CAD build for the part. Positions are in the model's coordinates, mm. A direction names the side the tool comes from. Coordinates: 2 decimals unless noted, no trailing zeros. Order: outer loops, then holes, each group sorted by start corner. A loop starts at its lowest first (then second) coordinate and runs counter-clockwise, first axis right, second up. Notation, with made-up numbers: M -24,73.25 L -19,73.25 A15 cw -19,99.25 Z; hole C 29.25,44.5 d1. An arc over 180 degrees is marked long. Write item = value, one per line.
Autodesk Inventor part; units mm, degrees
ref_plane "YZ Plane" through (0, 0, 0) normal (1, 0, 0) x (0, 1, 0)
ref_plane "XZ Plane" through (0, 0, 0) normal (0, 1, 0) x (-1, 0, 0)
ref_plane "XY Plane" through (0, 0, 0) normal (0, 0, 1) x (1, 0, 0)
sketch "Sketch1" plane through (0, 0, 0) normal (0, 1, 0) x (-1, 0, 0)
  line L0 (18, 20) -> (-18, 20)
  line L1 (-20, 18) -> (-20, -18)
  line L2 (-18, -20) -> (18, -20)
  line L3 (20, -18) -> (20, 18)
  line L4 (20, 20) -> (-20, -20) construction
  line L5 (-20, 20) -> (20, -20) construction
  circle A0 centre (0, 0) radius 11.5
  circle A1 centre (0, 0) radius 18.945
  arc A2 (20, 18) -> (18, 20) centre (18, 18) ccw
  arc A3 (18, -20) -> (20, -18) centre (18, -18) ccw
  arc A4 (-20, -18) -> (-18, -20) centre (-18, -18) ccw
  arc A5 (-18, 20) -> (-20, 18) centre (-18, 18) ccw
  dimension "d0" = 40
  dimension "d1" = 40
  dimension "d2" = 23
  dimension "d3" = 37.89
  dimension "d4" = 2
extrude "Extrusion1" add sketch "Sketch1" along normal blind 11
sketch "Sketch2" plane through (0, 0, 0) normal (0, -1, 0) x (1, 0, 0)
  line L0 (-20, -18) -> (-20, 18)
  arc A0 (-18, 20) -> (-20, 18) centre (-18, 18) ccw
  line L1 (-18, 20) -> (18, 20)
  arc A1 (20, 18) -> (18, 20) centre (18, 18) ccw
  line L2 (20, 18) -> (20, -18)
  arc A2 (18, -20) -> (20, -18) centre (18, -18) ccw
  line L3 (18, -20) -> (-18, -20)
  arc A3 (-20, -18) -> (-18, -20) centre (-18, -18) ccw
  point P0 (0, 0)
extrude "Extrusion2" add sketch "Sketch2" against normal blind 1
sketch "Sketch3" plane through (0, 11, 0) normal (0, 1, 0) x (1, 0, 0)
  circle A0 centre (0, 0) radius 11.5
  circle A1 centre (0, 0) radius 10.9
  dimension "d9" = 0.6
extrude "Extrusion3" cut sketch "Sketch3" against normal through all contours A1
sketch "Sketch4" plane through (0, 11, 0) normal (0, 1, 0) x (1, 0, 0)
  circle A0 centre (0, 0) radius 18.945 construction
  line L0 (-18, -20) -> (18, -20) construction
  arc A1 (18, -20) -> (20, -18) centre (18, -18) ccw construction
  line L1 (20, -18) -> (20, 18) construction
  arc A2 (20, 18) -> (18, 20) centre (18, 18) ccw construction
  line L2 (18, 20) -> (-18, 20) construction
  arc A3 (-18, 20) -> (-20, 18) centre (-18, 18) ccw construction
  line L3 (-20, 18) -> (-20, -18) construction
  arc A4 (-20, -18) -> (-18, -20) centre (-18, -18) ccw construction
  line L4 (-16.1, -16.1) -> (16.1, -16.1) construction
  line L5 (16.1, -16.1) -> (16.1, 16.1) construction
  line L6 (16.1, 16.1) -> (-16.1, 16.1) construction
  line L7 (-16.1, 16.1) -> (-16.1, -16.1) construction
  line L8 (-16.1, -16.1) -> (16.1, 16.1) construction
  line L9 (16.1, -16.1) -> (-16.1, 16.1) construction
  point P0 (0, 0)
  dimension "d12" = 32.2
  dimension "d13" = 32.2
hole "Hole1" at (-16.1, 11, 16.1) at (-16.1, 11, -16.1) at (16.1, 11, -16.1) at (16.1, 11, 16.1) direction (0, -1, 0) diameter 3.85 depth 10
sketch "Sketch14" plane through (20, 0, -18) normal (1, 0, 0) x (0, 0, -1)
  line L0 (0, 0) -> (0, 11) construction
  line L1 (-36, 11) -> (0, 11) construction
  line L2 (-36, 0) -> (-36, 11) construction
  line L3 (-36, 0) -> (0, 0) construction
  line L4 (-25.5, 10) -> (-10.5, 10)
  line L5 (-10.5, 10) -> (-10.5, 1)
  line L6 (-10.5, 1) -> (-25.5, 1)
  line L7 (-25.5, 1) -> (-25.5, 10)
  line L8 (-25.5, 10) -> (-10.5, 1) construction
  line L9 (-10.5, 10) -> (-25.5, 1) construction
  point P0 (-18, 0)
  point P1 (-18, 5.5)
  dimension "d47" = 15
  dimension "d48" = 9
extrude "Extrusion12" cut sketch "Sketch14" against normal blind 3
fillet "Fillet2" radius 2 2 edges at (17.3972, 5.5, 7.5) (17.3972, 5.5, -7.5)
sketch "Sketch15" plane through (0, 1, 0) normal (0, 1, 0) x (1, 0, 0)
  arc A0 (18.6666, -7.5) -> (16.8842, -8.5929) centre (18.6666, -9.5) ccw construction
  line L0 (20, -7.5) -> (18.6666, -7.5) construction
  line L1 (20, 7.5) -> (20, -7.5) construction
  line L2 (20, 7.5) -> (18.6666, 7.5) construction
  arc A1 (16.8842, 8.5929) -> (18.6666, 7.5) centre (18.6666, 9.5) ccw construction
  arc A2 (16.6035, -9.1235) -> (16.8842, -8.5929) centre (0, 0) ccw
  arc A3 (11.2223, -2.5118) -> (11.5, 0.0176) centre (0, 0) ccw
  arc A4 (11.5, 0.0176) -> (16.8842, -8.5929) centre (21.1006, 0.0323) ccw
  arc A5 (10.9, 0.0167) -> (16.6207, -9.1319) centre (21.1006, 0.0323) ccw
  dimension "d52" = 0.6
extrude "Extrusion13" add sketch "Sketch15" along normal up to surface (10 mm away)
sketch "Sketch16" plane through (20, 10, -7.5) normal (0, -1, 0) x (1, 0, 0)
  arc A0 (-3.1158, -1.0929) -> (-3.1158, 16.0929) centre (-20, 7.5) ccw
  arc A1 (-1.3334, 0) -> (-3.1158, -1.0929) centre (-1.3334, -2) ccw
  line L0 (0, 0) -> (-1.3334, 0)
  line L1 (0, 15) -> (0, 0)
  line L2 (0, 15) -> (-1.3334, 15)
  arc A2 (-3.1158, 16.0929) -> (-1.3334, 15) centre (-1.3334, 17) ccw
extrude "Extrusion14" add sketch "Sketch16" along normal up to surface (9 mm away)
sketch "Sketch17" plane through (20, 0, -18) normal (1, 0, 0) x (0, 0, -1)
  line L0 (0, 0) -> (0, 11) construction
  line L1 (-36, 11) -> (0, 11) construction
  line L2 (-36, 0) -> (-36, 11) construction
  line L3 (-36, 0) -> (0, 0) construction
  circle A0 centre (-17.9824, 5.5) radius 5.1
  point P0 (-18, 0)
  dimension "d57" = 10.2
extrude "Extrusion15" cut sketch "Sketch17" against normal blind 3
sketch "Sketch18" plane through (0, 11, 0) normal (0, 1, 0) x (1, 0, 0)
  line L0 (-18, -20) -> (18, -20)
  arc A0 (18, -20) -> (20, -18) centre (18, -18) ccw
  line L1 (20, -18) -> (20, 18)
  arc A1 (20, 18) -> (18, 20) centre (18, 18) ccw
  line L2 (18, 20) -> (-18, 20)
  arc A2 (-18, 20) -> (-20, 18) centre (-18, 18) ccw
  line L3 (-20, 18) -> (-20, -18)
  arc A3 (-20, -18) -> (-18, -20) centre (-18, -18) ccw
  circle A4 centre (16.1, -16.1) radius 1.925
  circle A5 centre (-16.1, 16.1) radius 1.925
  circle A6 centre (-16.1, -16.1) radius 1.925
  circle A7 centre (16.1, 16.1) radius 1.925
  circle A8 centre (0, 0) radius 10.9
  arc A9 (11.5, 0.0176) -> (11.2223, -2.5118) centre (0, 0) ccw
  arc A10 (11.2223, -2.5118) -> (16.6035, -9.1235) centre (21.1006, 0.0323) ccw
  arc A11 (16.8842, -8.5929) -> (16.6035, -9.1235) centre (0, 0) ccw
  arc A12 (11.5, 0.0176) -> (16.8842, -8.5929) centre (21.1006, 0.0323) ccw
extrude "Extrusion16" add sketch "Sketch18" along normal blind 1
sketch "Sketch19" plane through (0, 0, 0) normal (0, 1, 0) x (-1, 0, 0)
  arc A0 (-11.2223, 2.5118) -> (-16.6035, 9.1235) centre (-21.1006, -0.0323) ccw construction
  arc A1 (-16.8842, 8.5929) -> (-16.6035, 9.1235) centre (0, 0) ccw construction
  arc A2 (-11.5, -0.0176) -> (-16.8842, 8.5929) centre (-21.1006, -0.0323) ccw construction
  arc A3 (-11.5, -0.0176) -> (-11.2223, 2.5118) centre (0, 0) ccw construction
  circle A4 centre (0, 0) radius 10.9 construction
  circle A5 centre (-16.1, -16.1) radius 1.925 construction
  circle A6 centre (16.1, 16.1) radius 1.925 construction
  circle A7 centre (16.1, -16.1) radius 1.925 construction
  circle A8 centre (-16.1, 16.1) radius 1.925 construction
  line L0 (18, 20) -> (-18, 20) construction
  arc A9 (-18, 20) -> (-20, 18) centre (-18, 18) ccw construction
  line L1 (-20, 18) -> (-20, -18) construction
  arc A10 (-20, -18) -> (-18, -20) centre (-18, -18) ccw construction
  line L2 (-18, -20) -> (18, -20) construction
  arc A11 (18, -20) -> (20, -18) centre (18, -18) ccw construction
  line L3 (20, -18) -> (20, 18) construction
  arc A12 (20, 18) -> (18, 20) centre (18, 18) ccw construction
sketch "Sketch5" plane through (20, 0, -18) normal (1, 0, 0) x (0, 0, -1)
  line L0 (0, 0) -> (0, 11) construction
  line L1 (-36, 11) -> (0, 11) construction
  line L2 (-36, 0) -> (-36, 11) construction
  line L3 (-36, 0) -> (0, 0) construction
  line L4 (-20.5, 10) -> (-5.5, 10)
  line L5 (-5.5, 10) -> (-5.5, 1)
  line L6 (-5.5, 1) -> (-20.5, 1)
  line L7 (-20.5, 1) -> (-20.5, 10)
  line L8 (-20.5, 10) -> (-5.5, 1) construction
  line L9 (-5.5, 10) -> (-20.5, 1) construction
  point P0 (-18, 0)
  point P1 (-13, 5.5)
  dimension "d21" = 15
  dimension "d22" = 9
sketch "Sketch6" plane through (0, 1, 0) normal (0, 1, 0) x (1, 0, 0)
  line L0 (20, -2.5) -> (18.7339, -2.5) construction
  arc A0 (15.4996, 2.2947) -> (15.8884, 4.3911) centre (6.7587, 5) ccw
  arc A1 (15.8884, 4.3911) -> (18.7339, -2.5) centre (25.6093, 4.3721) ccw
  arc A2 (15.4996, 2.2947) -> (18.3979, -3.0115) centre (25.6093, 4.3721) ccw
  arc A3 (18.3979, -3.0115) -> (18.7339, -2.5) centre (6.7587, 5) ccw
  arc A4 (18.3979, -3.0115) -> (18.7339, -2.5) centre (6.7587, 5) ccw
  point P0 (0, 0)
  dimension "d25" = 0.6
sketch "Sketch12" plane through (20, 10, -12.5) normal (0, -1, 0) x (1, 0, 0)
  arc A0 (-4, 2.4397) -> (-1.2661, 15) centre (-20, 12.5) ccw
  line L0 (0, 0) -> (-4, 0)
  line L1 (0, 15) -> (0, 0)
  line L2 (0, 15) -> (-1.2661, 15)
  line L3 (-4, 2.4397) -> (-4, 0)
sketch "Sketch13" plane through (20, 0, -18) normal (1, 0, 0) x (0, 0, -1)
  line L0 (0, 0) -> (0, 11) construction
  line L1 (-36, 11) -> (0, 11) construction
  line L2 (-36, 0) -> (-36, 11) construction
  line L3 (-36, 0) -> (0, 0) construction
  circle A0 centre (-13, 5.5) radius 5.1
  point P0 (-18, 0)
  dimension "d44" = 10.2
sketch "Sketch8" plane through (20, 0, -13) normal (1, 0, 0) x (0, 0, -1)
  line L0 (-20.5, 10) -> (-5.5, 10)
  line L1 (-20.5, 1) -> (-20.5, 10)
  line L2 (-5.5, 1) -> (-20.5, 1)
  line L3 (-5.5, 10) -> (-5.5, 1)
  line L4 (-20.3, 9.8) -> (-5.7, 9.8)
  line L5 (-5.7, 9.8) -> (-5.7, 1.2)
  line L6 (-5.7, 1.2) -> (-20.3, 1.2)
  line L7 (-20.3, 1.2) -> (-20.3, 9.8)
  point P0 (-13, 0)
  dimension "d30" = 0.2
  dimension "d33" = 1
  dimension "d34" = 0.6
sketch "Sketch11" plane through (22.6, 0, -13) normal (1, 0, 0) x (0, 0, -1)
  line L0 (-21.3, 10.8) -> (-21.3, 0.2) construction
  line L1 (-21.3, 0.2) -> (-4.7, 0.2) construction
  line L2 (-4.7, 0.2) -> (-4.7, 10.8) construction
  line L3 (-4.7, 10.8) -> (-21.3, 10.8) construction
  circle A0 centre (-13, 5.5) radius 5.125
  point P0 (-13, 0)
  dimension "d39" = 10.25
properties part number "base3"
(1) Slice it at B-B, the plane y = 9.25. Write the cut outline in (x, z) (3 decimals).
Evaluation:
outline = M -20,-18 A2 ccw -18,-20 L 18,-20 A2 ccw 20,-18 L 20,-3.474 L 18.624,-3.474 A18.945 cw long 16.603,9.123 A10.201 ccw 11.222,2.512 A11.5 ccw long 11.5,-0.018 A9.601 cw 16.884,8.593 A18.945 cw 18.63,3.439 L 20,3.439 L 20,18 A2 ccw 18,20 L -18,20 A2 ccw -20,18 Z; hole C -16.1,-16.1 d3.85; hole C -16.1,16.1 d3.85; hole C 0,0 d21.8; hole C 16.1,-16.1 d3.85; hole C 16.1,16.1 d3.85
(2) Wall check: line 1 (X direction, y = 4.75, z = 0) (3 decimals); line 2 (X direction, y = 4, z = 9); line 3 (X direction, y = 8.5, z = 7.5). Give the ranges that are in metal, low to high. Write a range as from..to.
Evaluation:
line_1 = -20..-18.945, -11.5..-10.9, 10.9..11.5
line_2 = -20..-16.67, -7.16..-6.15, 6.15..7.16, 16.36..20
line_3 = -20..-17.4, -8.72..-7.91, 7.91..8.72, 14.22..15.15, 17.4..20
(3) Pull direction X, two halves, no side cores. Call faces 4 (the face through (-19.4, 5.92, 19.43)), 5 (the face through (19.4, 5.92, -19.43)), 6 (the face through (-5, 12, -10)), 7 (the face through (-17.116, 6.423, 17.735)): +X half, -X half, draft (parallel to the pull), parting line (faces both ways), or undercut.
Evaluation:
face_4 = -X half
face_5 = +X half
face_6 = draft
face_7 = undercut
(4) Pin check, flat tips, straight feed: pin 1 Ø1.2 at (x, z) = (-16, -15.5) entering from +Y; pin 2 Ø0.7 at (y, z) = (1, 0.5) entering from +X. Stop position of each tip, or through.
Evaluation:
pin_1 = 1
pin_2 = 17
(5) Tool access for faces 1 (the face through (20, 9, 4)), 2 (the face through (-17.117, 5.93, -8.118)), 3 (the face through (18.85, 0.52, 1.09)): list every direction of +Z, -Z, +X, -X, +Y, -Y with a clear straight run to the whole face (end or side of a thin tool).
Evaluation:
face_1 = +Z, -Z, +X, +Y, -Y
face_2 = +Y
face_3 = +X
(6) Slice it at A-A, the plane x = -7. Write the cut outline in (y, z), then the cut area to 3 significant figures.
Evaluation:
outline = M 0,-20 L 12,-20 L 12,-17.6 L 1,-17.6 L 1,-9.12 L 12,-9.12 L 12,-8.36 L 0,-8.36 Z; M 0,8.36 L 12,8.36 L 12,9.12 L 1,9.12 L 1,17.6 L 12,17.6 L 12,20 L 0,20 Z
area = 92.9 mm²
